Check sheet for the modelled part. Datum: model origin and axes. Units: mm. Round coordinates to 2 decimals unless told otherwise and drop trailing zeros. Loops run counter-clockwise (first coordinate to the right, second up) from the corner with the lowest first, then second, coordinate; pieces in that order, holes last. Notation, with made-up numbers: (75.25, 40) - (121.25, 40) arc R17 ccw to (121.25, 47) - close; hole circle Ø9 at (47, 77.5). An arc over 180 degrees is marked (long way). Put each result on its own line as item: value. Start each with the question number.
Item 1: Material ranges on line 1 along Y through (x, z) = (0, 8.25); line 2 along X through (y, z) = (-150, 10); line 3 along Y through (x, z) = (-1, 11.75), recorded low to high.
Item 2: Section check B-B, the plane z = 10. Record the cut outline in (x, y).
Item 3: Section check A-A, the plane x = 0. Record the cut outline in (y, z).
Item 4: Gauge pin test, flat ends, axial feed: pin 1 Ø4 at (x, z) = (10, 9.5) entering from -Y; pin 2 Ø8 at (x, y) = (0, -150) entering from -Z; pin 3 Ø5 at (x, z) = (-5, 13.5) entering from +Y; pin 4 Ø10 at (x, y) = (4.5, 64.5) entering from -Z. Record the tip position at first contact, or that the pin passes through.
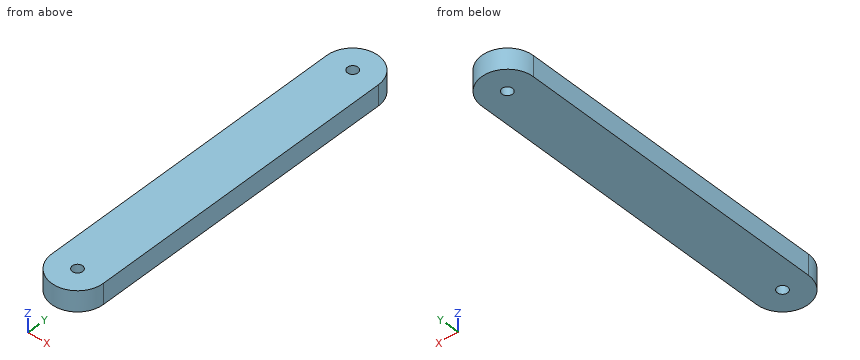
Autodesk Inventor part; units mm, degrees
ref_plane "YZ Plane" through (0, 0, 0) normal (1, 0, 0) x (0, 1, 0)
ref_plane "XZ Plane" through (0, 0, 0) normal (0, 1, 0) x (-1, 0, 0)
ref_plane "XY Plane" through (0, 0, 0) normal (0, 0, 1) x (1, 0, 0)
sketch "Sketch1" plane through (0, 0, 0) normal (0, 0, 1) x (1, 0, 0)
  line L0 (-7.5, 170) -> (7.5, 170)
  line L1 (7.5, 170) -> (7.5, -170)
  line L2 (7.5, -170) -> (-7.5, -170)
  line L3 (-7.5, -170) -> (-7.5, 170)
  line L4 (-10.5, 0) -> (10.5, 0)
  line L5 (0, -238) -> (0, 238)
  point P0 (0, 0)
  dimension "d4" = 7.5
  dimension "d5" = 7.5
  dimension "d6" = 170
  dimension "d7" = 170
extrude "Extrusion1" add sketch "Sketch1" along normal blind 20
sketch "Sketch2" plane through (0, 0, 20) normal (0, 0, 1) x (1, 0, 0)
  circle A0 centre (0, 150) radius 5
  circle A1 centre (0, -150) radius 5
  line L0 (-10.5, 0) -> (10.5, 0)
  line L1 (0, -238) -> (0, 238)
  point P0 (0, 0)
  dimension "d8" = 10
  dimension "d9" = 150
  dimension "d10" = 150
  dimension "d11" = 10
extrude "Extrusion2" cut sketch "Sketch2" against normal blind 180
sketch "Sketch3" plane through (0, 0, 20) normal (0, 0, 1) x (1, 0, 0)
  arc A0 (25, 149.8188) -> (-25, 149.8188) centre (0, 149.8188) ccw
  circle A1 centre (0, -150) radius 5
  arc A2 (-25, -150) -> (25, -150) centre (0, -150) ccw
  line L0 (-25, 149.8188) -> (-25, -150)
  line L1 (25, 149.8188) -> (25, -150)
  line L2 (7.5, -170) -> (7.5, 170)
  point P0 (0, 0)
  dimension "d12" = 50
  dimension "d13" = 50
extrude "Extrusion3" add sketch "Sketch3" against normal blind 20
mirror "Mirror1" about plane through (0, 0, 0) normal (0, 1, 0) of "Extrusion2"
Check result:
1. line 1: -175 to -155, -145 to 145, 155 to 174.82
1. line 2: -25 to -5, 5 to 25
1. line 3: -174.98 to -154.9, -145.1 to 145.1, 154.9 to 174.8
2. outline: (-25, -150) arc R25 ccw to (25, -150) - (25, 149.82) arc R25 ccw to (-25, 149.82) - close; hole circle Ø10 at (0, -150); hole circle Ø10 at (0, 150)
3. outline: (-175, 0) - (-155, 0) - (-155, 20) - (-175, 20) - close; (-145, 0) - (145, 0) - (145, 20) - (-145, 20) - close; (155, 0) - (174.82, 0) - (174.82, 20) - (155, 20) - close
4. pin 1: y = -173.69
4. pin 2: through
4. pin 3: y = 174.69
4. pin 4: z = 0
